from build123d import *

# Parameters (mm, degrees)
BOSS_EXTRUDE1_DEPTH = 6.35
SKETCH3_R           = 2.032
CUT_EXTRUDE1_DEPTH  = 80.985269666


with BuildPart() as part:
    # Sketch1 → Boss-Extrude1 (new body)
    with BuildSketch(Plane.XY):
        with BuildLine():
            Line((-10.998522628, 6.35), (-26.121491239, -19.843749996))
            ThreePointArc((-26.121491239, -19.843749996), (-27.390226605, -22.906748123), (-27.822968611, -26.193749996))
            Line((-27.822968611, -26.193749996), (-27.822968611, -32.702820897))
            Line((-27.822968611, -32.702820897), (-44.45, -55.598546415))
            Line((-44.45, -55.598546415), (-57.15, -55.598546415))
            Line((-57.15, -55.598546415), (-57.15, 23.954310777))
            Line((-57.15, 23.954310777), (15.615566787, 23.954310777))
            Line((15.615566787, 23.954310777), (33.111768772, -6.35))
            Line((33.111768772, -6.35), (18.330871047, -6.35))
            Line((18.330871047, -6.35), (10.998522628, 6.35))
            ThreePointArc((10.998522628, 6.35), (0, 12.7), (-10.998522628, 6.35))
        make_face()
    extrude(amount=BOSS_EXTRUDE1_DEPTH)

    # Sketch3 → Cut-Extrude1 (cut, through all)
    with BuildSketch(Plane.XY.offset(6.35)):
        with Locations((-50.8, -49.248546415)):
            Circle(SKETCH3_R)
    extrude(amount=-CUT_EXTRUDE1_DEPTH, mode=Mode.SUBTRACT)


solid = part.part
Model file for the job. Use its own axes, mm. A direction names the side the tool comes from. Round coordinates to 2 decimals unless told otherwise and drop trailing zeros. Loops run counter-clockwise (first coordinate to the right, second up) from the corner with the lowest first, then second, coordinate; pieces in that order, holes last. Notation, with made-up numbers: (-22, -25.75) -> (1, -25.75) arc R22 cw to (1, 0.25) -> close; hole circle Ø6 at (13, 55). An arc over 180 degrees is marked (long way). Answer as CSV lines item,"result". Start each with the question number.
1) Pin check, flat tips, straight feed: P1, Ø12, axis at x = -4, y = -3, coming from the -Z side; P2, Ø3, axis at x = 25.5, z = 2, coming from the -Y side. Stop position of each tip, or through.
2) Tool access for faces 1 (the face through (-27.823, -29, 3)), 2 (the face through (-57.15, -16, 3)), 3 (the face through (-18.45, -6.56, 3.13)): list every direction of +Z, -Z, +X, -X, +Y, -Y with a clear straight run to the whole face (end or side of a thin tool).
3) Mould opens along X. For faces 4 (the face through (-31, -6, 0)), 5 (the face through (24.241, 9.014, 3.131)), 6 (the face through (-52.3, -47.88, 3.22)) say: +X half, -X half, draft (parallel to the pull), parting line (faces both ways), or undercut.
4) Slice it at B-B (y = -2.5). List the corners of the cut face in (x, z), plus the area to 3 significant figures.
5) Probe line 1 along Y through (x, z) = (-50.8, 2.5); line 2 along X through (y, z) = (10, 1); line 3 along X through (y, z) = (11, 4). List the from-to ranges inside material, lowest first.
6) Slice it at A-A (x = -50.8). List the corners of the cut face in (y, z), plus the area to 3 significant figures.
7) Slice it at D-D (y = -10.5). List the corners of the cut face in (x, z), plus the area to 3 significant figures.
8) Slice it at C-C (z = 5). List the corners of the cut face in (x, y).
Filled in:
1,P1,"passes through"
1,P2,"stops at y = -6.35"
2,face 1,"+Z, -Z, +X, -Y"
2,face 2,"+Z, -Z, -X, +Y, -Y"
2,face 3,"+Z, -Z, -Y"
3,face 4,"draft"
3,face 5,"+X half"
3,face 6,"undercut"
4,outline,"(-57.15, 0) -> (-16.11, 0) -> (-16.11, 6.35) -> (-57.15, 6.35) -> close; (16.11, 0) -> (30.89, 0) -> (30.89, 6.35) -> (16.11, 6.35) -> close"
4,area,"354 mm2"
5,line 1,"y = -55.6 to -51.28, -47.22 to 23.95"
5,line 2,"x = -57.15 to -7.83, 7.83 to 23.67"
5,line 3,"x = -57.15 to -6.35, 6.35 to 23.09"
6,outline,"(-55.6, 0) -> (-51.28, 0) -> (-51.28, 6.35) -> (-55.6, 6.35) -> close; (-47.22, 0) -> (23.95, 0) -> (23.95, 6.35) -> (-47.22, 6.35) -> close"
6,area,"479 mm2"
7,outline,"(-57.15, 0) -> (-20.73, 0) -> (-20.73, 6.35) -> (-57.15, 6.35) -> close"
7,area,"231 mm2"
8,outline,"(-57.15, -55.6) -> (-44.45, -55.6) -> (-27.82, -32.7) -> (-27.82, -26.19) arc R12.7 cw to (-26.12, -19.84) -> (-11, 6.35) arc R12.7 cw to (11, 6.35) -> (18.33, -6.35) -> (33.11, -6.35) -> (15.62, 23.95) -> (-57.15, 23.95) -> close; hole circle Ø4.06 at (-50.8, -49.25)"
